Job drawing, mm, ordinate dimensions from the low corner. One solid piece. Give positions to 0.01 mm unless a question says otherwise; leave off trailing zeros. Loops run counter-clockwise (first coordinate to the right, second up) from the corner with the lowest first, then second, coordinate; pieces in that order, holes last. Notation, with made-up numbers: (70.25, 41) -> (106.25, 41) arc R19 ccw to (106.25, 75) -> close; hole circle Ø9 at (13, -10.5). An arc over 180 degrees is marked (long way). Answer as a JSON object with one key per item and string values. Group by question number.
Q1. Wall check: probe 1 along Y at (x, z) = (31.75, 11); probe 2 along Z at (x, y) = (2, 14.5); probe 3 along X at (y, z) = (10.5, 16.25). Give the ranges that are in metal, low to high. Write a range as from..to.
Q2. Band-saw the part on C-C, the plane z = 11.75. Write the cut outline in (x, y), plus the area to 3 significant figures.
Q3. Two-plate mould, pull along Y, no slides. Class the marked faces 1, 2 and 3: pulls with the +Y half, pulls with the -Y half, needs draft (parallel to the pull), parting line crosses it, or undercut.
Q4. Band-saw the part on D-D, the plane x = 8.5. Write the cut outline in (y, z).
Q5. Band-saw the part on B-B, the plane y = 18. Write the cut outline in (x, z), plus the area to 3 significant figures.
Q6. Drop flat-ended pins along their axis: pin 1 (2 mm diameter, centred on y = 16, z = 9.5, fed in from -X); pin 2 (1.5 mm diameter, centred on x = 28.5, z = 2.5, fed in from -Y); pin 3 (5 mm diameter, centred on y = 7.5, z = 16.5, fed in from -X). Give the stop position or say it passes through.
Q7. Band-saw the part on A-A, the plane x = 29.5. Write the cut outline in (y, z).
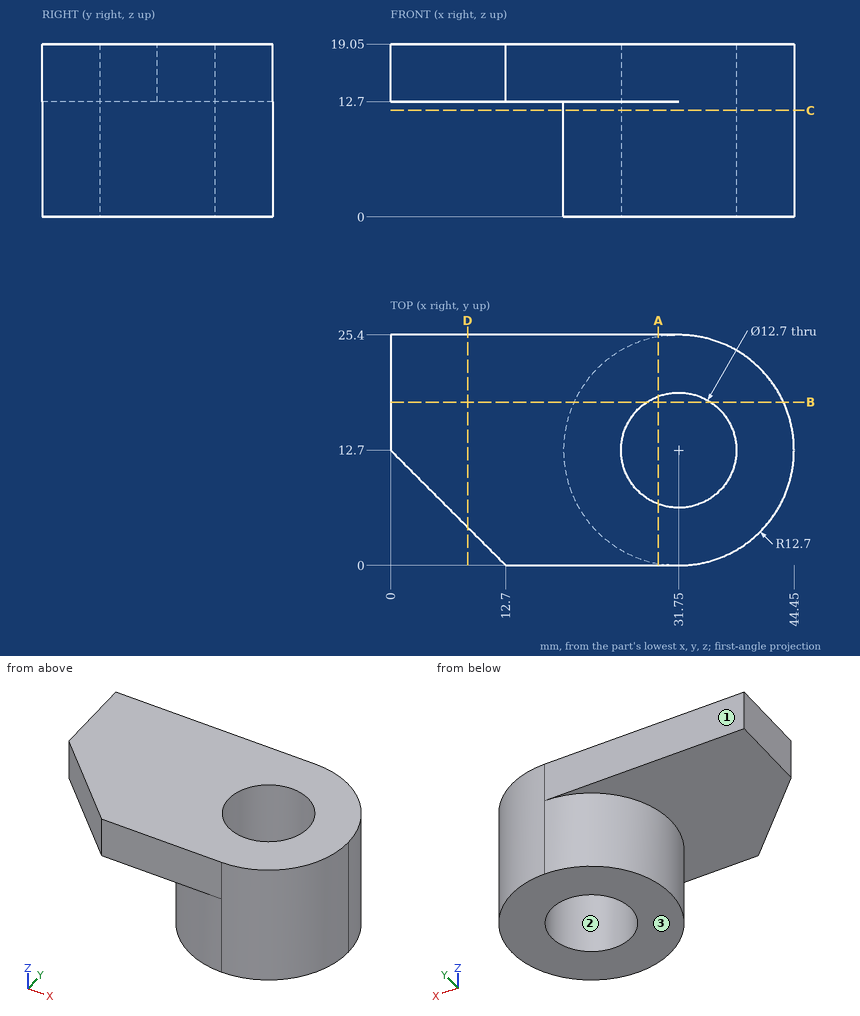
Worked answers:
{
 "1": {"probe 1": "0..6.35, 19.05..25.4", "probe 2": "12.7..19.05", "probe 3": "2.2..25.79, 37.71..44.26"},
 "2": {"outline": "circle Ø25.4 at (31.75, 12.7); hole circle Ø12.7 at (31.75, 12.7)", "area": "380 mm2"},
 "3": {"face 1": "pulls with the +Y half", "face 2": "undercut", "face 3": "needs draft"},
 "4": {"outline": "(4.2, 12.7) -> (25.4, 12.7) -> (25.4, 19.05) -> (4.2, 19.05) -> close"},
 "5": {"outline": "(0, 12.7) -> (20.21, 12.7) -> (20.21, 0) -> (28.25, 0) -> (28.25, 19.05) -> (0, 19.05) -> close; (35.25, 0) -> (43.29, 0) -> (43.29, 19.05) -> (35.25, 19.05) -> close", "area": "435 mm2"},
 "6": {"pin 1": "x = 19.26", "pin 2": "y = 0.25", "pin 3": "x = 2.7"},
 "7": {"outline": "(0, 12.7) -> (0.2, 12.7) -> (0.2, 0) -> (6.76, 0) -> (6.76, 19.05) -> (0, 19.05) -> close; (18.64, 0) -> (25.2, 0) -> (25.2, 12.7) -> (25.4, 12.7) -> (25.4, 19.05) -> (18.64, 19.05) -> close"}
}
